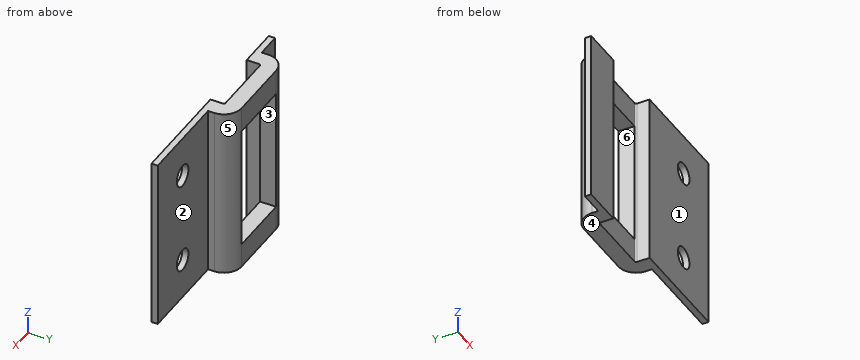
Autodesk Inventor part; units mm, degrees
ref_plane "YZ Plane" through (0, 0, 0) normal (1, 0, 0) x (0, 1, 0)
ref_plane "XZ Plane" through (0, 0, 0) normal (0, 1, 0) x (-1, 0, 0)
ref_plane "XY Plane" through (0, 0, 0) normal (0, 0, 1) x (1, 0, 0)
sketch "Sketch1" plane through (0, 0, 0) normal (0, 0, 1) x (1, 0, 0)
  line L0 (-5.575, 0) -> (6.925, 0)
  line L1 (6.925, 2.35) -> (6.925, 0)
  line L2 (-5.575, 2.35) -> (-5.575, 0)
  line L3 (-5.275, 2.65) -> (6.625, 2.65)
  arc A0 (-5.275, 2.65) -> (-5.575, 2.35) centre (-5.275, 2.35) ccw
  arc A1 (6.925, 2.35) -> (6.625, 2.65) centre (6.625, 2.35) ccw
  line L4 (-5.575, 0) -> (6.925, 0)
  line L5 (-8.575, 0) -> (-8.575, 2.35)
  arc A2 (-5.275, 5.65) -> (-8.575, 2.35) centre (-5.275, 2.35) ccw
  line L6 (-5.275, 5.65) -> (6.625, 5.65)
  arc A3 (9.925, 2.35) -> (6.625, 5.65) centre (6.625, 2.35) ccw
  line L7 (9.925, 2.35) -> (9.925, 0)
  line L8 (-8.575, 0) -> (9.925, 0)
  line L9 (6.925, 1.175) -> (14.545, 1.175)
  line L10 (14.545, 1.175) -> (14.545, 0)
  line L11 (14.545, 0) -> (6.925, 0)
  line L12 (6.925, 1.175) -> (6.925, 0)
  line L13 (-5.575, 1.175) -> (-13.195, 1.175)
  line L14 (-5.575, 1.175) -> (2.045, 1.175) construction
  line L15 (-13.195, 1.175) -> (-13.195, 0)
  line L16 (-13.195, 0) -> (14.545, 0)
  point P0 (0, 0)
  point P1 (-8.575, 1.175)
  point P2 (-5.275, 2.65)
  point P3 (9.925, 1.175)
  dimension "d0" = 3
  dimension "d1" = 3
  dimension "d2" = 7.62
  dimension "d3" = 7.62
  dimension "d4" = 180
extrude "Extrusion1" add sketch "Sketch1" along normal blind 32.0548 contours L8 L5 L13 L2 | L1 L9 L7 L8 | L13 L5 A2 L6 A3 L7 L9 L1 A1 L3 A0 L2 | L16 L15 L13 L5 | L7 L9 L10 L11
sketch "Sketch2" plane through (-5.275, 5.65, 0) normal (0, 1, 0) x (1, 0, 0)
  line L0 (0, -32.0548) -> (11.9, -32.0548)
  line L1 (5.95, -32.0548) -> (5.95, -15.939)
  line L2 (0, 0) -> (0, -32.0548)
  line L3 (0, -4.509) -> (11.9, -4.509)
  line L4 (11.9, -4.509) -> (11.9, -27.369)
  line L5 (11.9, -27.369) -> (0, -27.369)
  line L6 (0, -27.369) -> (0, -4.509)
  line L7 (0, -4.509) -> (11.9, -27.369) construction
  line L8 (11.9, -4.509) -> (0, -27.369) construction
  line L9 (11.9, 0) -> (0, 0)
  dimension "d7" = 22.86
extrude "Extrusion2" cut sketch "Sketch2" against normal blind 32.0548 contours L2 L3 L4 L5
sketch "Sketch3" plane through (14.545, 0, 0) normal (1, 0, 0) x (0, 0, -1)
  line L0 (0, 0) -> (0, 1.175)
  line L1 (0, 1.175) -> (-32.0548, 1.175)
  line L2 (-32.0548, 0) -> (-32.0548, 1.175)
  line L3 (0, 0) -> (-32.0548, 0)
extrude "Extrusion3" add sketch "Sketch3" along normal blind 12.7
sketch "Sketch4" plane through (9.925, 1.175, 32.0548) normal (0, 1, 0) x (1, 0, 0)
  line L0 (0, 32.0548) -> (17.32, 32.0548)
  line L1 (0, 32.0548) -> (0, 0)
  line L2 (0, 0) -> (17.32, 0)
  line L3 (17.32, 32.0548) -> (17.32, 0)
  line L4 (0, 0) -> (8.7376, 0)
  line L5 (-3, 0) -> (17.32, 0)
  line L6 (8.7376, 0) -> (8.7376, 7.5184)
  circle A0 centre (8.7376, 7.5184) radius 2
  line L7 (0, 32.0548) -> (8.7376, 32.0548)
  line L8 (-3, 32.0548) -> (17.32, 32.0548)
  line L9 (8.7376, 32.0548) -> (8.7376, 24.5364)
  circle A1 centre (8.7376, 24.5364) radius 2
  point P0 (-9.925, 32.0548)
  dimension "d12" = 8.7376
  dimension "d13" = 7.5184
  dimension "d14" = 4
  dimension "d15" = 8.7376
  dimension "d16" = 7.5184
  dimension "d17" = 90
  dimension "d18" = 4
extrude "Extrusion4" cut sketch "Sketch4" against normal up to surface (1.175 mm away) contours A0 | A1
properties part number "Servo Holder Cap"
Geometry check sheet. Reference: the model listing, model coordinates, mm. Face numbers are marked on the shaded views. A direction names the side the tool comes from. Give positions to 0.01 mm unless a question says otherwise; leave off trailing zeros. Order: outer loops, then holes, each group sorted by start corner. A loop starts at its lowest first (then second) coordinate and runs counter-clockwise, first axis right, second up.
1. Section check B-B, the plane x = -4. Enter the section's corners in (y, z).
2. Section check D-D, the plane z = 29.5. Enter the section's corners in (x, y) (3 decimals).
3. Section check C-C, the plane y = 4.2. Enter the section's corners in (x, z) (3 decimals).
4. Access from +Z, -Z, +X, -X, +Y, -Y to the whole of each face (thin tool, end or side, straight path). Record for the marked faces 1 and 2.
5. Thickness scan on L1, parallel to X at y = 0.85, z = 18 (3 decimals); L2, parallel to X at y = 2.3, z = 10 (3 decimals); L3, parallel to Z at x = 1.5, y = 3.4. Record the ranges inside material, lowest first.
6. Release check for a two-part mould opening along Z. For the marked faces 3, 4, 5 and 6 record: pulls with the +Z half, pulls with the -Z half, needs draft (parallel to the pull), parting line crosses it, or undercut.
7. Gauge pin test, flat ends, axial feed: pin 1 Ø0.9 at (y, z) = (3.5, 15) entering from -X; pin 2 Ø2.5 at (x, z) = (-0.5, 29) entering from -Y; pin 3 Ø1.5 at (y, z) = (4.5, 14) entering from +X. Record the tip position at first contact, or that the pin passes through.
8. Section check A-A, the plane z = 17. Enter the section's corners in (x, y) (3 decimals), and give its area (3 significant figures).
Values follow:
1. outline: (2.65, 0) - (5.65, 0) - (5.65, 4.51) - (2.65, 4.51) - close; (2.65, 27.37) - (5.65, 27.37) - (5.65, 32.05) - (2.65, 32.05) - close
2. outline: (-13.195, 0) - (-5.575, 0) - (-5.575, 2.35) arc R0.3 cw to (-5.275, 2.65) - (6.625, 2.65) arc R0.3 cw to (6.925, 2.35) - (6.925, 0) - (27.245, 0) - (27.245, 1.175) - (9.925, 1.175) - (9.925, 2.35) arc R3.3 ccw to (6.625, 5.65) - (-5.275, 5.65) arc R3.3 ccw to (-8.575, 2.35) - (-8.575, 1.175) - (-13.195, 1.175) - close
3. outline: (-8.008, 0) - (9.358, 0) - (9.358, 32.055) - (-8.008, 32.055) - close; hole (-5.275, 4.509) - (6.625, 4.509) - (6.625, 27.369) - (-5.275, 27.369) - close
4. face 1: +Z, -Z, +X, -X, -Y
4. face 2: +Z, -Z, +X, +Y
5. L1: x = -13.195 to -5.575, 6.925 to 27.245
5. L2: x = -8.575 to -5.575, 6.925 to 9.925
5. L3: z = 0 to 4.51, 27.37 to 32.05
6. face 3: undercut
6. face 4: pulls with the -Z half
6. face 5: needs draft
6. face 6: undercut
7. pin 1: stops at x = -8.5
7. pin 2: stops at y = 2.65
7. pin 3: stops at x = 9.61
8. outline: (-13.195, 0) - (-5.575, 0) - (-5.575, 2.35) arc R0.3 cw to (-5.275, 2.65) - (-5.275, 5.65) arc R3.3 ccw to (-8.575, 2.35) - (-8.575, 1.175) - (-13.195, 1.175) - close; (6.625, 2.65) arc R0.3 cw to (6.925, 2.35) - (6.925, 0) - (27.245, 0) - (27.245, 1.175) - (9.925, 1.175) - (9.925, 2.35) arc R3.3 ccw to (6.625, 5.65) - close
8. area: 56.8 mm2
